```python
from build123d import *

# Parameters (mm, degrees)
CONG_1_R                                           = 2.5
ENL_V_MAT_EXTRU_1_REACH                            = 181.165
CHAMBRAGE_POUR_VIS_T_TE_HEXAGONALE_M16_D           = 17.5
CHAMBRAGE_POUR_VIS_T_TE_HEXAGONALE_M16_DEPTH       = 20
CHAMBRAGE_POUR_VIS_T_TE_HEXAGONALE_M16_CBORE_D     = 26
CHAMBRAGE_POUR_VIS_T_TE_HEXAGONALE_M16_CBORE_DEPTH = 16.6
CHAMBRAGE_POUR_VIS_T_TE_HEXAGONALE_M16_TIP         = 5.257530416
ECHELLE1_SCALE                                     = 0.25


with BuildPart() as part:
    # Esquisse1 → Révolution1 (revolve)
    with BuildSketch(Plane.XY, mode=Mode.PRIVATE) as r_volution1_sk:
        with BuildLine():
            Line((0, 0), (80, 0))
            Line((80, 0), (80, 20))
            Line((80, 20), (23.203122076, 20))
            ThreePointArc((23.203122076, 20), (22.035240729, 14.861087101), (20, 10))
            Line((20, 10), (0, 10))
            Line((0, 10), (0, 0))
        make_face()
    revolve(r_volution1_sk.sketch.rotate(Axis((80, 20, 0), (0, -1, 0)), 270), axis=Axis((80, 20, 0), (0, -1, 0)))

    # Congé1
    cong_1_edges = [part.edges().sort_by_distance(p)[0] for p in [
        (80, 10, -80),
        (80, 20, -56.796877924),
        (80, 0, -80),
    ]]
    fillet(cong_1_edges, radius=CONG_1_R)

    # Esquisse3 → Enlèv. mat.-Extru.1 (cut, up to next)
    with BuildSketch(Plane(origin=(0, 10, 0), x_dir=(1, 0, 0), z_dir=(0, 1, 0)), mode=Mode.PRIVATE) as enl_v_mat_extru_1_sk1:
        with BuildLine():
            Line((0.001700291, 0.521578063), (70.517699728, 79.436049635))
            ThreePointArc((70.517699728, 79.436049635), (20.346266679, 53.305085132), (0.001700291, 0.521578063))
        make_face()
    enl_v_mat_extru_1_tool1 = extrude(enl_v_mat_extru_1_sk1.sketch, amount=-ENL_V_MAT_EXTRU_1_REACH, mode=Mode.PRIVATE) & part.part
    add(enl_v_mat_extru_1_tool1.solids().sort_by_distance((29.225405, 10, -45.370909))[0], mode=Mode.SUBTRACT)

    # Chambrage pour vis à tête hexagonale M161
    with Locations(Plane(origin=(0, 20, 0), x_dir=(1, 0, 0), z_dir=(0, 1, 0))):
        with Locations((79.591089576, 0)):
            CounterBoreHole(CHAMBRAGE_POUR_VIS_T_TE_HEXAGONALE_M16_D / 2, CHAMBRAGE_POUR_VIS_T_TE_HEXAGONALE_M16_CBORE_D / 2, CHAMBRAGE_POUR_VIS_T_TE_HEXAGONALE_M16_CBORE_DEPTH, depth=CHAMBRAGE_POUR_VIS_T_TE_HEXAGONALE_M16_DEPTH)
            with Locations((0, 0, -(CHAMBRAGE_POUR_VIS_T_TE_HEXAGONALE_M16_DEPTH + CHAMBRAGE_POUR_VIS_T_TE_HEXAGONALE_M16_TIP / 2))):  # 118° drill point
                Cone(0, CHAMBRAGE_POUR_VIS_T_TE_HEXAGONALE_M16_D / 2, CHAMBRAGE_POUR_VIS_T_TE_HEXAGONALE_M16_TIP, mode=Mode.SUBTRACT)


with BuildPart() as part_1:
    # Echelle1: scaled about (82.57091432, 8.513984125, 2.2848071)
    add(part.part.scale(ECHELLE1_SCALE).moved(Location((61.92818574, 6.385488094, 1.713605325))))


solid = part_1.part
```
Can you work these out from the model? Positions are in its coordinate system, mm. A direction names the side the tool comes from. Give positions to 0.01 mm unless a question says otherwise; leave off trailing zeros. Write each loop counter-clockwise with the first axis right and the second up, starting at its lowest first coordinate (ties: lowest second). Pieces come first, ordered by that corner, then holes. Notation, with made-up numbers: (25, -23) - (44, -23) arc R29 ccw to (44, 16) - close; hole circle Ø3 at (-5, -13.5). An arc over 180 degrees is marked (long way). Write item = value, one per line. Start each with the question number.
1. Please list where these lines run through material, in increasing order: line 1 (Z direction, x = 85.5, y = 8.8); line 2 (Y direction, x = 92.5, z = -13.5); line 3 (Z direction, x = 80.5, y = 7.7).
2. On a 3-axis mill with a long thin cutter (end or side, diameter ignored), from which of +Z, -Z, +X, -X, +Y, -Y can I reach the whole of each face in a straight line? I mean faces 5 (the face through (95, 8.885, 10)), 6 (the face through (79.74, 6.8, 1.06)). Say none if no direction works.
3. Imagine slicing it at A-A (y = 10.05). Please give me the cut outline in (x, z).
4. Thinking about a two-plate mould opening in X: for faces 1 (the face through (83, 7.235, 4)), 2 (the face through (97.28, 7.63, 14.53)), 3 (the face through (70.62, 7.653, -8.143)), 4 (the face through (86, 6.385, 1)), which applies, released by +X, released by -X, zero draft, split by the parting line, or undercut?
5. For pin 1 (1.5 mm diameter, centred on x = 70, y = 7.5, fed in from +Z); pin 2 (1 mm diameter, centred on x = 90, z = 16.5, fed in from +Y); pin 3 (1 mm diameter, centred on x = 74, y = 10, fed in from +Z); pin 4 (3.5 mm diameter, centred on x = 81.83, z = 1.71, fed in from +Y), each with a flat end and sliding along its axis, tell me the tip position at first contact or that it passes through.
Worked answers:
q1.line_1 = -17.65 to 21.08
q1.line_2 = 6.39 to 8.89
q1.line_3 = -18.24 to -1.25, 4.68 to 21.66
q2.face_5 = +Y
q2.face_6 = +Y, -Y
q3.outline = circle Ø29.02 at (81.93, 1.71); hole circle Ø6.5 at (81.83, 1.71)
q4.face_1 = undercut
q4.face_2 = split by the parting line
q4.face_3 = released by -X
q4.face_4 = zero draft
q5.pin_1 = 18.3
q5.pin_2 = 8.89
q5.pin_3 = 14.26
q5.pin_4 = through
